from build123d import *

# Parameters (mm, degrees)
SKETCH1_W                       = 165.1
SKETCH1_H                       = 101.6
BOSS_EXTRUDE1_DEPTH             = 254
CUT_EXTRUDE1_DEPTH              = 254
SKETCH5_R                       = 20.447
BOSS_EXTRUDE3_DEPTH             = 139.7
BOSS_EXTRUDE3_DIRECTION_2_REACH = 285.127
SHELL2_T                        = -2.54


with BuildPart() as part:
    # Sketch1 → Boss-Extrude1 (new body)
    with BuildSketch(Plane(origin=(0, 0, 0), x_dir=(1, 0, 0), z_dir=(0, 1, 0))):
        Rectangle(SKETCH1_W, SKETCH1_H)
    extrude(amount=BOSS_EXTRUDE1_DEPTH)

    # Sketch2 → Cut-Extrude1 (cut)
    with BuildSketch(Plane(origin=(0, 0, -50.8), x_dir=(-1, 0, 0), z_dir=(0, 0, -1))):
        Polygon((-44.45, 0), (-82.55, 25.4), (-82.55, 0), align=None)
    extrude(amount=-CUT_EXTRUDE1_DEPTH, mode=Mode.SUBTRACT)

    # Sketch5 → Boss-Extrude3 (add)
    with BuildSketch(Plane(origin=(31.75, 254, 0), x_dir=(0.9657919899307167, -0.2399824072752947, 0.09825617733263003), z_dir=(0.2588190451025181, 0.8685657757104482, -0.422618261740697))):
        with Locations(Location((0, 0, 0), (0, 0, 269.046198917))):
            Circle(SKETCH5_R)
    extrude(amount=BOSS_EXTRUDE3_DEPTH)

    # Boss-Extrude3 direction 2: up to this face of the body (flat: up to its plane)
    boss_extrude3_direction_2_end = Plane(part.part.faces().sort_by_distance((0, 254, 0))[0])
    # Sketch5 → Boss-Extrude3 direction 2 (add, up to the picked face)
    with BuildSketch(Plane(origin=(31.75, 254, 0), x_dir=(0.9657919899307167, -0.2399824072752947, 0.09825617733263003), z_dir=(0.2588190451025181, 0.8685657757104482, -0.422618261740697)), mode=Mode.PRIVATE) as boss_extrude3_direction_2_sk1:
        with Locations(Location((0, 0, 0), (0, 0, 269.046198917))):
            Circle(SKETCH5_R)
    boss_extrude3_direction_2_tool1 = split(extrude(boss_extrude3_direction_2_sk1.sketch, amount=-BOSS_EXTRUDE3_DIRECTION_2_REACH, mode=Mode.PRIVATE), bisect_by=boss_extrude3_direction_2_end, keep=Keep.BOTH, mode=Mode.PRIVATE)
    add(boss_extrude3_direction_2_tool1.solids().sort_by(Axis((31.75, 254, 0), (-0.2588190451025181, -0.8685657757104482, 0.422618261740697)))[0])

    # Shell2
    shell2_openings = [part.faces().sort_by_distance(p)[0] for p in [
        (67.907020601, 375.338638867, -59.039771165),
    ]]
    offset(amount=SHELL2_T, openings=shell2_openings, kind=Kind.INTERSECTION)


solid = part.part
The listing builds one solid part. Answer for the finished solid, in the listing's coordinates (mm). A direction names the side the tool comes from. Give positions to 0.01 mm unless a question says otherwise; leave off trailing zeros. Order: outer loops, then holes, each group sorted by start corner. A loop starts at its lowest first (then second) coordinate and runs counter-clockwise, first axis right, second up. Notation, with made-up numbers: (4, 0) - (28, 0) arc R5 ccw to (28, 5) - close; hole circle Ø9 at (82, 31.5). An arc over 180 degrees is marked (long way). Use one line per item in the form item = value.
1) The mould has two halves that part along Y. Classify faces 4 (the flat face through (82.55, 138, 1)), 5 (the flat face through (80.01, 138, 1)), 6 (the flat face through (50.443, 379.505, -61.173)): released by +Y, released by -Y, zero draft, split by the parting line, or undercut.
Verdict:
face_4 = zero draft
face_5 = undercut
face_6 = released by +Y
2) Find section A-A on x = -35. Determine the outline of the cut face in (y, z).
Verdict:
outline = (0, -50.8) - (254, -50.8) - (254, 50.8) - (0, 50.8) - close; hole (2.54, -48.26) - (251.46, -48.26) - (251.46, 48.26) - (2.54, 48.26) - close
3) Consider probe 1 along Y at (x, z) = (-15, -29); probe 2 along Z at (x, y) = (14, 18); probe 3 along X at (y, z) = (239.5, -34). Determine where each line is inside the solid, lowest interval first. Write a range as [from, to].
Verdict:
probe_1 = [0, 2.54], [251.46, 254]
probe_2 = [-50.8, -48.26], [48.26, 50.8]
probe_3 = [-82.55, -80.01], [80.01, 82.55]
4) Find section C-C on z = 36. Determine the outline of the cut face in (x, y), and give its area (3 significant figures).
Verdict:
outline = (-82.55, 0) - (44.45, 0) - (82.55, 25.4) - (82.55, 254) - (-82.55, 254) - close; hole (-80.01, 2.54) - (43.68, 2.54) - (80.01, 26.76) - (80.01, 251.46) - (-80.01, 251.46) - close
area = 2,060 mm^2
5) For faces 1 (the flat face through (63.2, 12.5, -0.7)), 2 (the flat face through (-80.01, 125, 1)), 3 (the flat face through (-1, 125, -50.8)), determine the directions among +Z, -Z, +X, -X, +Y, -Y from which every point of the face is accessible in a straight line to the end or side of a thin tool.
Verdict:
face_1 = +Z, -Z, +X, -Y
face_2 = none
face_3 = -Z, +X, -X, -Y
6) Each of these flat-tipped pins is pushed along its axis until it touches: pin 1 (10 mm diameter, centred on x = -20.5, y = 93.5, fed in from -Z); pin 2 (12 mm diameter, centred on y = 194, z = -8, fed in from +X); pin 3 (3 mm diameter, centred on x = -30.5, z = -23, fed in from +Y). Where does it stop, or does it pass through?
Verdict:
pin_1 = -50.8
pin_2 = 82.55
pin_3 = 254
7) Find section B-B on y = 205. Determine the outline of the cut face in (x, z), and give its area (3 significant figures).
Verdict:
outline = (-82.55, -50.8) - (82.55, -50.8) - (82.55, 50.8) - (-82.55, 50.8) - close; hole (-80.01, -48.26) - (80.01, -48.26) - (80.01, 48.26) - (-80.01, 48.26) - close
area = 1,330 mm^2
